```python
from build123d import *

# Parameters (mm, degrees)
SKETCH_1_W          = 20
SKETCH_1_H          = 16
SKETCH_1_R          = 2.5
EXTRUDE_1_DEPTH     = 1
SKETCH_2_W          = 1
SKETCH_2_H          = 16
EXTRUDE_2_DEPTH     = 19
SKETCH_3_R          = 2.5
CUT_EXTRUDE_1_DEPTH = 32.890437438
FILLET_2_R          = 2


with BuildPart() as part:
    # 草图1 → 凸台-拉伸1 (new body)
    with BuildSketch(Plane.XY):
        with Locations((10, 8)):
            Rectangle(SKETCH_1_W, SKETCH_1_H)
        with Locations((5.5, 10.5)):
            Circle(SKETCH_1_R, mode=Mode.SUBTRACT)
        with Locations((12.5, 5.5)):
            Circle(SKETCH_1_R, mode=Mode.SUBTRACT)
    extrude(amount=EXTRUDE_1_DEPTH)

    # 草图2 → 凸台-拉伸2 (add)
    with BuildSketch(Plane.XY.offset(1)):
        with Locations((19.5, 8)):
            Rectangle(SKETCH_2_W, SKETCH_2_H)
    extrude(amount=EXTRUDE_2_DEPTH)

    # 草图3 → 切除-拉伸1 (cut, through all)
    with BuildSketch(Plane.ZY.offset(-19)):
        with Locations(Location((7.5, 10.5, 0), (0, 0, 270))):
            Circle(SKETCH_3_R)
        with Locations(Location((14.5, 5.5, 0), (0, 0, 270))):
            Circle(SKETCH_3_R)
    extrude(amount=-CUT_EXTRUDE_1_DEPTH, mode=Mode.SUBTRACT)

    # 圆角2
    fillet_2_edges = [part.edges().sort_by_distance(p)[0] for p in [
        (19, 8, 1),
        (20, 8, 0),
    ]]
    fillet(fillet_2_edges, radius=FILLET_2_R)


solid = part.part
```
The listing builds one solid part. Answer for the finished solid, in the listing's coordinates (mm). A direction names the side the tool comes from. Round coordinates to 2 decimals unless told otherwise and drop trailing zeros. Write each loop counter-clockwise with the first axis right and the second up, starting at its lowest first coordinate (ties: lowest second). Pieces come first, ordered by that corner, then holes. Notation, with made-up numbers: (-33.5, -35) -> (-8.5, -35) arc R12 ccw to (-8.5, -22) -> close; hole circle Ø10 at (-17, 49.25). An arc over 180 degrees is marked (long way). Answer as a JSON object with one key per item and string values. Group by question number.
Q1. Section A-A (y = 3.5) is taken. Write down the section's boundary in (x, z).
Q2. Section D-D (y = 9) is taken. Write down the section's boundary in (x, z), plus the area to 3 significant figures.
Q3. Straight lines are drawn through the part: line 1 along Y through (x, z) = (12.5, 0.55); line 2 along Z through (x, y) = (16.25, 11.5); line 3 along Y through (x, z) = (5.5, 0.25). For each, find the intervals that lie inside material, in ascending order.
Q4. Each of these flat-tipped pins is pushed along its axis until it touches: pin 1 Ø6 at (y, z) = (10.5, 7.5) entering from -X; pin 2 Ø5 at (x, y) = (5, 3) entering from +Z; pin 3 Ø8 at (x, z) = (8.5, 2.5) entering from -Y. Where does it stop, or does it pass through?
Q5. Which of the six approach directions +Z, -Z, +X, -X, +Y, -Y give full straight-line access (tool end or side, diameter ignored) to faces 1 (the face through (19.5, 8.1, 20)), 2 (the face through (8, 8, 1))?
Q6. Determine the mould class of faces 3 (the face through (15.1, 0, 0.3)), 4 (the face through (19.49, 4.35, 12.28)), 5 (the face through (20, 8, 11)) for opening direction Y: pulls with the +Y half, pulls with the -Y half, needs draft (parallel to the pull), parting line crosses it, or undercut.
Q7. Section C-C (x = 5.5) is taken. Write down the section's boundary in (y, z), plus the area to 3 significant figures.
Q8. Section B-B (z = 7.5) is taken. Write down the section's boundary in (x, y), plus the area to 3 significant figures.
Check values:
{
 "1": {"outline": "(0, 0) -> (11, 0) -> (11, 1) -> (0, 1) -> close; (14, 0) -> (18, 0) arc R2 ccw to (20, 2) -> (20, 13) -> (19, 13) -> (19, 3) arc R2 cw to (17, 1) -> (14, 1) -> close; (19, 16) -> (20, 16) -> (20, 20) -> (19, 20) -> close"},
 "2": {"outline": "(0, 0) -> (3.5, 0) -> (3.5, 1) -> (0, 1) -> close; (7.5, 0) -> (18, 0) arc R2 ccw to (20, 2) -> (20, 5.5) -> (19, 5.5) -> (19, 3) arc R2 cw to (17, 1) -> (7.5, 1) -> close; (19, 9.5) -> (20, 9.5) -> (20, 20) -> (19, 20) -> close", "area": "31.0 mm^2"},
 "3": {"line 1": "0 to 3, 8 to 16", "line 2": "0 to 1", "line 3": "0 to 8, 13 to 16"},
 "4": {"pin 1": "x = 19", "pin 2": "z = 1", "pin 3": "y = 0"},
 "5": {"face 1": "+Z, +X, -X, +Y, -Y", "face 2": "+Z, -X, +Y, -Y"},
 "6": {"face 3": "pulls with the -Y half", "face 4": "undercut", "face 5": "needs draft"},
 "7": {"outline": "(0, 0) -> (8, 0) -> (8, 1) -> (0, 1) -> close; (13, 0) -> (16, 0) -> (16, 1) -> (13, 1) -> close", "area": "11.0 mm^2"},
 "8": {"outline": "(19, 0) -> (20, 0) -> (20, 8) -> (19, 8) -> close; (19, 13) -> (20, 13) -> (20, 16) -> (19, 16) -> close", "area": "11.0 mm^2"}
}
